Here's how the part is built. I have some questions about the finished solid (model axes, mm). A direction names the side the tool comes from. Coordinates: 2 decimals unless noted, no trailing zeros. Loops run counter-clockwise (first coordinate to the right, second up) from the corner with the lowest first, then second, coordinate; pieces in that order, holes last. Notation, with made-up numbers: (59, 41) -> (83, 41) arc R37 ccw to (83, 80) -> close; hole circle Ø9 at (-34.5, -38). An arc over 180 degrees is marked (long way). Answer as a JSON object with one key per item and string values. Group by question number.
Q1. I want a section at C-C on x = 26. Write out the boundary of the cut face in (y, z), then the cut area to 3 significant figures.
Q2. I want a section at B-B on y = 0. Write out the boundary of the cut face in (x, z), then the cut area to 3 significant figures.
Q3. I need wall thicknesses on line 1 (Y direction, x = 38, z = 104); line 2 (Y direction, x = 4.25, z = 0) (3 decimals); line 3 (Z direction, x = 40, y = -112.25). Which ranges of each line are inside material? Lowest first, please.
Q4. I want a section at D-D on z = 17.5. Write out the boundary of the cut face in (x, y).
Q5. Thinking about a two-plate mould opening in Y: for faces 1 (the flat face through (11, 130, -9)), 2 (the cylindrical face through (7.605, 69.528, -77.604)), 3 (the conical face through (39.503, -99.51, 97.394)), which applies, released by +Y, released by -Y, zero draft, split by the parting line, or undercut?
Q6. I'm going to push flat-ended pins straight in: pin 1 (9.5 mm diameter, centred on x = 40, z = 97.55, fed in from +Y); pin 2 (6 mm diameter, centred on x = 38, y = 61, fed in from +Z); pin 3 (1 mm diameter, centred on y = -44.5, z = 61, fed in from -X); pin 4 (0.6 mm diameter, centred on y = 116, z = -136, fed in from -X). Where does each tip first touch, or does it pass through?
Q7. I want a section at A-A on z = 107.5. Write out the boundary of the cut face in (x, y), then the cut area to 3 significant figures.
Q8. On a 3-axis mill with a long thin cutter (end or side, diameter ignored), from which of +Z, -Z, +X, -X, +Y, -Y can I reach the whole of each face in a straight line? I mean faces 4 (the flat face through (11, -2, -150)), 5 (the cylindrical face through (20.706, -3.964, -90.063)), 6 (the cylindrical face through (39.15, 98.07, 98.34)). Say none if no direction works.
```python
from build123d import *

# Parameters (mm, degrees)
SKETCH1_W                  = 300
SKETCH1_H                  = 260
BOSS_EXTRUDE1_DEPTH        = 60.5
SKETCH2_R                  = 90.15
CUT_EXTRUDE1_DEPTH         = 42
SKETCH9_R                  = 41.51
CUT_EXTRUDE9_DEPTH         = 306
SKETCH12_W                 = 39
SKETCH12_H                 = 260
CUT_EXTRUDE12_DEPTH        = 36.45
SKETCH13_W                 = 39
SKETCH13_H                 = 260
CUT_EXTRUDE13_DEPTH        = 14
SKETCH14_W                 = 39
SKETCH14_H                 = 249.55
CUT_EXTRUDE14_DEPTH        = 14
SKETCH15_W                 = 22.45
SKETCH15_H                 = 260
CUT_EXTRUDE15_DEPTH        = 208.50963833
F_6_0MM_DOWEL_HOLE1_D      = 6
F_6_0MM_DOWEL_HOLE1_DEPTH  = 30
F_6_0MM_DOWEL_HOLE1_TIP    = 1.802581857
F_6_0MM_DOWEL_HOLE2_D      = 6
F_6_0MM_DOWEL_HOLE2_DEPTH  = 30
F_6_0MM_DOWEL_HOLE2_TIP    = 1.802581857
F_6_0MM_DOWEL_HOLE3_D      = 6
F_6_0MM_DOWEL_HOLE3_DEPTH  = 15
F_6_0MM_DOWEL_HOLE3_TIP    = 1.802581857
SKETCH25_W                 = 39
SKETCH25_H                 = 14
CUT_EXTRUDE16_DEPTH        = 313.400788251
SKETCH26_W                 = 257.55
SKETCH26_H                 = 240
CUT_EXTRUDE17_DEPTH        = 2.3
F_10_0MM_DOWEL_HOLE1_D     = 10
F_10_0MM_DOWEL_HOLE1_DEPTH = 15
F_10_0MM_DOWEL_HOLE1_TIP   = 3.004303095
SKETCH31_R                 = 95.65
SKETCH31_R_2               = 91.65
CUT_EXTRUDE18_DEPTH        = 2.3
SKETCH32_R                 = 2.25
CUT_EXTRUDE19_DEPTH        = 68


with BuildPart() as part:
    # Sketch1 → Boss-Extrude1 (new body)
    with BuildSketch(Plane(origin=(0, 0, 0), x_dir=(0, 0, -1), z_dir=(1, 0, 0))):
        Rectangle(SKETCH1_W, SKETCH1_H)
    extrude(amount=BOSS_EXTRUDE1_DEPTH)

    # Sketch2 → Cut-Extrude1 (cut)
    with BuildSketch(Plane(origin=(0, 0, 0), x_dir=(0, 0, -1), z_dir=(1, 0, 0))):
        with Locations(Location((0, 0, 0), (0, 0, 180))):
            Circle(SKETCH2_R)
    extrude(amount=CUT_EXTRUDE1_DEPTH, mode=Mode.SUBTRACT)

    # Sketch9 → Cut-Extrude9 (cut)
    with BuildSketch(Plane(origin=(0, 0, 0), x_dir=(0, 0, -1), z_dir=(1, 0, 0))):
        with Locations(Location((0, 0, 0), (0, 0, 180))):
            Circle(SKETCH9_R)
    extrude(amount=CUT_EXTRUDE9_DEPTH, mode=Mode.SUBTRACT)

    # Sketch12 → Cut-Extrude12 (cut)
    with BuildSketch(Plane.XY.offset(150)):
        with Locations((41, 0)):
            Rectangle(SKETCH12_W, SKETCH12_H)
    extrude(amount=-CUT_EXTRUDE12_DEPTH, mode=Mode.SUBTRACT)

    # Sketch13 → Cut-Extrude13 (cut)
    with BuildSketch(Plane(origin=(0, 0, -150), x_dir=(-1, 0, 0), z_dir=(0, 0, -1))):
        with Locations((-41, 0)):
            Rectangle(SKETCH13_W, SKETCH13_H)
    extrude(amount=-CUT_EXTRUDE13_DEPTH, mode=Mode.SUBTRACT)

    # Sketch14 → Cut-Extrude14 (cut)
    with BuildSketch(Plane(origin=(0, -130, 0), x_dir=(-1, 0, 0), z_dir=(0, -1, 0))):
        with Locations((-41, 11.225)):
            Rectangle(SKETCH14_W, SKETCH14_H)
    extrude(amount=-CUT_EXTRUDE14_DEPTH, mode=Mode.SUBTRACT)

    # Sketch15 → Cut-Extrude15 (cut, through all)
    with BuildSketch(Plane(origin=(0, 0, 0), x_dir=(0, 0, -1), z_dir=(1, 0, 0))):
        with Locations((-138.775, 0)):
            Rectangle(SKETCH15_W, SKETCH15_H)
    extrude(amount=CUT_EXTRUDE15_DEPTH, mode=Mode.SUBTRACT)

    # Ø6.0mm Dowel Hole1
    with Locations(Plane(origin=(0, 0, -136), x_dir=(-1, 0, 0), z_dir=(0, 0, -1))):
        with Locations((-38.5, 101), (-38.5, -76)):
            Hole(F_6_0MM_DOWEL_HOLE1_D / 2, depth=F_6_0MM_DOWEL_HOLE1_DEPTH)
            with Locations((0, 0, -(F_6_0MM_DOWEL_HOLE1_DEPTH + F_6_0MM_DOWEL_HOLE1_TIP / 2))):  # 118° drill point
                Cone(0, F_6_0MM_DOWEL_HOLE1_D / 2, F_6_0MM_DOWEL_HOLE1_TIP, mode=Mode.SUBTRACT)

    # Ø6.0mm Dowel Hole2
    with Locations(Plane.XY.offset(113.55)):
        with Locations((38.5, 101), (38.5, -76)):
            Hole(F_6_0MM_DOWEL_HOLE2_D / 2, depth=F_6_0MM_DOWEL_HOLE2_DEPTH)
            with Locations((0, 0, -(F_6_0MM_DOWEL_HOLE2_DEPTH + F_6_0MM_DOWEL_HOLE2_TIP / 2))):  # 118° drill point
                Cone(0, F_6_0MM_DOWEL_HOLE2_D / 2, F_6_0MM_DOWEL_HOLE2_TIP, mode=Mode.SUBTRACT)

    # Ø6.0mm Dowel Hole3
    with Locations(Plane(origin=(0, -116, 0), x_dir=(-1, 0, 0), z_dir=(0, -1, 0))):
        with Locations((-40, -97.55), (-40, 120)):
            Hole(F_6_0MM_DOWEL_HOLE3_D / 2, depth=F_6_0MM_DOWEL_HOLE3_DEPTH)
            with Locations((0, 0, -(F_6_0MM_DOWEL_HOLE3_DEPTH + F_6_0MM_DOWEL_HOLE3_TIP / 2))):  # 118° drill point
                Cone(0, F_6_0MM_DOWEL_HOLE3_D / 2, F_6_0MM_DOWEL_HOLE3_TIP, mode=Mode.SUBTRACT)

    # Sketch25 → Cut-Extrude16 (cut, through all)
    with BuildSketch(Plane(origin=(0, 0, -150), x_dir=(-1, 0, 0), z_dir=(0, 0, -1))):
        with Locations((-41, 123)):
            Rectangle(SKETCH25_W, SKETCH25_H)
    extrude(amount=-CUT_EXTRUDE16_DEPTH, mode=Mode.SUBTRACT)

    # Sketch26 → Cut-Extrude17 (cut)
    with BuildSketch(Plane(origin=(21.5, 0, 0), x_dir=(0, 0, -1), z_dir=(1, 0, 0))):
        with Locations((11.225, 0)):
            Rectangle(SKETCH26_W, SKETCH26_H)
        with BuildLine():
            Line((-113.05, 116), (135.5, 116))
            ThreePointArc((135.5, 116), (135.853553391, 115.853553391), (136, 115.5))
            Line((136, 115.5), (136, -115.5))
            ThreePointArc((136, -115.5), (135.853553391, -115.853553391), (135.5, -116))
            Line((135.5, -116), (-113.05, -116))
            ThreePointArc((-113.05, -116), (-113.403553391, -115.853553391), (-113.55, -115.5))
            Line((-113.55, -115.5), (-113.55, 115.5))
            ThreePointArc((-113.55, 115.5), (-113.403553391, 115.853553391), (-113.05, 116))
        make_face(mode=Mode.SUBTRACT)
    extrude(amount=-CUT_EXTRUDE17_DEPTH, mode=Mode.SUBTRACT)

    # Ø10.0mm Dowel Hole1
    with Locations(Plane.ZY):
        with Locations((-82.598742079, 69.308574014), (0, 107.825), (82.598742079, 69.308574014), (82.598742079, -69.308574014), (0, -107.825), (-82.598742079, -69.308574014)):
            Hole(F_10_0MM_DOWEL_HOLE1_D / 2, depth=F_10_0MM_DOWEL_HOLE1_DEPTH)
            with Locations((0, 0, -(F_10_0MM_DOWEL_HOLE1_DEPTH + F_10_0MM_DOWEL_HOLE1_TIP / 2))):  # 118° drill point
                Cone(0, F_10_0MM_DOWEL_HOLE1_D / 2, F_10_0MM_DOWEL_HOLE1_TIP, mode=Mode.SUBTRACT)

    # Sketch31 → Cut-Extrude18 (cut)
    with BuildSketch(Plane(origin=(0, 0, 0), x_dir=(0, 0, -1), z_dir=(1, 0, 0))):
        Circle(SKETCH31_R)
        Circle(SKETCH31_R_2, mode=Mode.SUBTRACT)
    extrude(amount=CUT_EXTRUDE18_DEPTH, mode=Mode.SUBTRACT)

    # Sketch32 → Cut-Extrude19 (cut)
    with BuildSketch(Plane(origin=(0, -130, 0), x_dir=(-1, 0, 0), z_dir=(0, -1, 0))):
        with Locations(Location((-9, 9.45, 0), (0, 0, 90))):
            Circle(SKETCH32_R)
    extrude(amount=-CUT_EXTRUDE19_DEPTH, mode=Mode.SUBTRACT)


solid = part.part
```
Result set:
{
 "1": {"outline": "(-116, -136) -> (116, -136) -> (116, 113.55) -> (-116, 113.55) -> close; hole circle Ø180.3 at (0, 0)", "area": "32,400 mm²"},
 "2": {"outline": "(0, -150) -> (21.5, -150) -> (21.5, -140) -> (19.2, -140) -> (19.2, -136) -> (60.5, -136) -> (60.5, -41.51) -> (42, -41.51) -> (42, -90.15) -> (0, -90.15) -> (0, -91.65) -> (2.3, -91.65) -> (2.3, -95.65) -> (0, -95.65) -> close; (0, 90.15) -> (42, 90.15) -> (42, 41.51) -> (60.5, 41.51) -> (60.5, 113.55) -> (19.2, 113.55) -> (19.2, 117.55) -> (21.5, 117.55) -> (21.5, 127.55) -> (0, 127.55) -> (0, 95.65) -> (2.3, 95.65) -> (2.3, 91.65) -> (0, 91.65) -> close", "area": "6,550 mm²"},
 "3": {"line 1": "y = -116 to -78.96, -73.04 to 98.04, 103.96 to 116", "line 2": "y = -130 to -112.825, -102.825 to -90.15, 90.15 to 102.825, 112.825 to 130", "line 3": "z = -136 to -123, -117 to 94.55, 100.55 to 113.55"},
 "4": {"outline": "(0, -130) -> (21.5, -130) -> (21.5, -120) -> (19.2, -120) -> (19.2, -116) -> (60.5, -116) -> (60.5, -37.64) -> (42, -37.64) -> (42, -88.44) -> (0, -88.44) -> (0, -89.96) -> (2.3, -89.96) -> (2.3, -94.04) -> (0, -94.04) -> close; (0, 88.44) -> (42, 88.44) -> (42, 37.64) -> (60.5, 37.64) -> (60.5, 116) -> (19.2, 116) -> (19.2, 120) -> (21.5, 120) -> (21.5, 130) -> (0, 130) -> (0, 94.04) -> (2.3, 94.04) -> (2.3, 89.96) -> (0, 89.96) -> close"},
 "5": {"face 1": "released by +Y", "face 2": "undercut", "face 3": "released by -Y"},
 "6": {"pin 1": "stops at y = 116", "pin 2": "stops at z = 113.55", "pin 3": "stops at x = 42", "pin 4": "stops at x = 0"},
 "7": {"outline": "(0, -130) -> (21.5, -130) -> (21.5, -120) -> (19.2, -120) -> (19.2, -116) -> (60.5, -116) -> (60.5, 116) -> (19.2, 116) -> (19.2, 120) -> (21.5, 120) -> (21.5, 130) -> (0, 130) -> close; hole circle Ø6 at (38.5, -76); hole circle Ø6 at (38.5, 101)", "area": "14,600 mm²"},
 "8": {"face 4": "-Z, +X, -X, +Y, -Y", "face 5": "-X", "face 6": "+Z"}
}
